Model file for the job. Use its own axes, mm. Round coordinates to 2 decimals unless told otherwise and drop trailing zeros. Loops run counter-clockwise (first coordinate to the right, second up) from the corner with the lowest first, then second, coordinate; pieces in that order, holes last. Notation, with made-up numbers: (63, 3.5) -> (103, 3.5) arc R22 cw to (103, 30.5) -> close; hole circle Ø3 at (14, 35.25). An arc over 180 degrees is marked (long way). Use a Markdown table: item, result. Add a question column.
```python
from build123d import *

# Parameters (mm, degrees)
F1_DEPTH = 10


with BuildPart() as f1:
    # F0 (on Right) → F1 (new body)
    with BuildSketch(Plane.YZ):
        with BuildLine():
            Line((115.396181, 316.925998), (-1.603819, 316.925998))
            Line((-1.603819, 316.925998), (-1.603819, 6.925998))
            Line((-1.603819, 6.925998), (-21.603819, 6.925998))
            Line((-21.603819, 6.925998), (-21.603819, -3.074002))
            Line((-21.603819, -3.074002), (-1.603819, -3.074002))
            Line((-1.603819, -3.074002), (-1.603819, -13.074002))
            Line((-1.603819, -13.074002), (-21.603819, -13.074002))
            Line((-21.603819, -13.074002), (-21.603819, -23.074002))
            Line((-21.603819, -23.074002), (-1.603819, -23.074002))
            Line((-1.603819, -23.074002), (-1.603819, -73.074002))
            Line((-1.603819, -73.074002), (-21.603819, -73.074002))
            Line((-21.603819, -73.074002), (-21.603819, -83.074002))
            Line((-21.603819, -83.074002), (-1.603819, -83.074002))
            Line((-1.603819, -83.074002), (-1.603819, -93.074002))
            Line((-1.603819, -93.074002), (-21.603819, -93.074002))
            Line((-21.603819, -93.074002), (-21.603819, -103.074002))
            Line((-21.603819, -103.074002), (-1.603819, -103.074002))
            Line((-1.603819, -103.074002), (-1.603819, -153.074002))
            Line((-1.603819, -153.074002), (-21.603819, -153.074002))
            Line((-21.603819, -153.074002), (-21.603819, -143.074002))
            Line((-21.603819, -143.074002), (-31.603819, -143.074002))
            Line((-31.603819, -143.074002), (-31.603819, -163.074002))
            Line((-31.603819, -163.074002), (-1.603819, -163.074002))
            Line((-1.603819, -163.074002), (-1.603819, -203.074002))
            Line((-1.603819, -203.074002), (-4.103819, -203.074002))
            ThreePointArc((-4.103819, -203.074002), (-6.603819, -204.415689), (-9.103819, -203.074002))
            Line((-9.103819, -203.074002), (-14.103819, -203.074002))
            ThreePointArc((-14.103819, -203.074002), (-16.603819, -204.415689), (-19.103819, -203.074002))
            Line((-19.103819, -203.074002), (-21.603819, -203.074002))
            Line((-21.603819, -203.074002), (-21.603819, -213.074002))
            Line((-21.603819, -213.074002), (8.396181, -213.074002))
            Line((8.396181, -213.074002), (8.396181, 306.925998))
            Line((8.396181, 306.925998), (105.396181, 306.925998))
            Line((105.396181, 306.925998), (105.396181, 281.925998))
            Line((105.396181, 281.925998), (115.396181, 281.925998))
            Line((115.396181, 281.925998), (115.396181, 316.925998))
        make_face()
    extrude(amount=-F1_DEPTH)


solid = f1.part
```
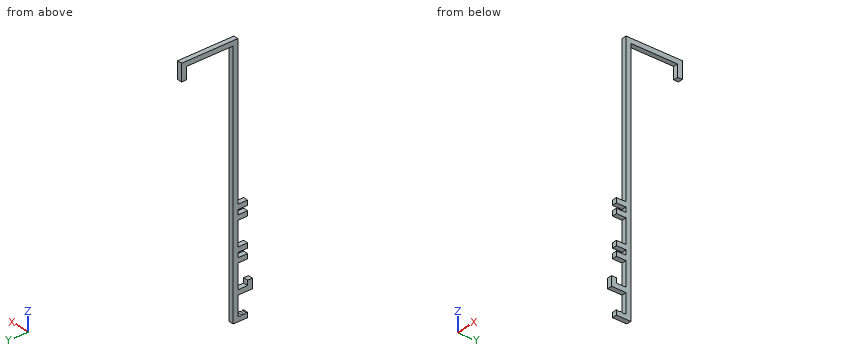
1) Pin check, flat tips, straight feed: pin 1 Ø3 at (x, z) = (-5, -8.5) entering from -Y; pin 2 Ø3 at (x, y) = (-5, -20) entering from +Z; pin 3 Ø2 at (x, y) = (-3, 88) entering from -Z. Stop position of each tip, or through.
2) Cut at B-B on z = -65.5. Write the cut outline in (x, y), and give its area (3 significant figures).
3) Cut at A-A on y = 17.5. Write the cut outline in (x, z).
4) Wall check: probe 1 along Z at (x, y) = (-1.5, -12.5); probe 2 along Z at (x, y) = (-9, -6); probe 3 along Y at (x, z) = (-2.25, 285.5). Give the ranges that are in metal, low to high. Write a range as from..to.
Established:
| question | item | result |
|---|---|---|
| 1 | pin 1 | stops at y = -1.6 |
| 1 | pin 2 | stops at z = 6.93 |
| 1 | pin 3 | stops at z = 306.93 |
| 2 | outline | (-10, -1.6) -> (0, -1.6) -> (0, 8.4) -> (-10, 8.4) -> close |
| 2 | area | 100 mm^2 |
| 3 | outline | (-10, 306.93) -> (0, 306.93) -> (0, 316.93) -> (-10, 316.93) -> close |
| 4 | probe 1 | z = -213.07..-203.07, -163.07..-153.07, -103.07..-93.07, -83.07..-73.07, -23.07..-13.07, -3.07..6.93 |
| 4 | probe 2 | z = -213.07..-204.35, -163.07..-153.07, -103.07..-93.07, -83.07..-73.07, -23.07..-13.07, -3.07..6.93 |
| 4 | probe 3 | y = -1.6..8.4, 105.4..115.4 |
